```python
from build123d import *

# Parameters (mm, degrees)
SKETCH1_R           = 40
BOSS_EXTRUDE1_DEPTH = 25
SKETCH2_R           = 38
CUT_EXTRUDE1_DEPTH  = 2
SKETCH3_R           = 37
CUT_EXTRUDE2_DEPTH  = 21.5
SKETCH4_W           = 12.5
SKETCH4_H           = 11.5
CUT_EXTRUDE3_DEPTH  = 41
SKETCH5_R           = 1.05
CUT_EXTRUDE4_DEPTH  = 24
SKETCH6_W           = 4.251934594
SKETCH6_H           = 15.745280186
CUT_EXTRUDE5_DEPTH  = 1.2
SKETCH7_R           = 3.3
SKETCH7_R_2         = 1.5
BOSS_EXTRUDE2_DEPTH = 2.8
FILLET1_R           = 1
SKETCH9_R           = 4.75
SKETCH9_R_2         = 3.25
BOSS_EXTRUDE3_DEPTH = 6.4
SKETCH10_R          = 8
SKETCH10_R_2        = 3
BOSS_EXTRUDE4_DEPTH = 15.5
FILLET3_R           = 4


with BuildPart() as part:
    # Sketch1 → Boss-Extrude1 (new body)
    with BuildSketch(Plane(origin=(0, 0, 0), x_dir=(1, 0, 0), z_dir=(0, 1, 0))):
        with Locations(Location((0, 0, 0), (0, 0, 270))):  # turned: the seam where the file's is
            Circle(SKETCH1_R)
    extrude(amount=-BOSS_EXTRUDE1_DEPTH)

    # Sketch2 → Cut-Extrude1 (cut)
    with BuildSketch(Plane(origin=(0, 0, 0), x_dir=(1, 0, 0), z_dir=(0, 1, 0))):
        with Locations(Location((0, 0, 0), (0, 0, 270))):  # turned: the seam where the file's is
            Circle(SKETCH2_R)
    extrude(amount=-CUT_EXTRUDE1_DEPTH, mode=Mode.SUBTRACT)

    # Sketch3 → Cut-Extrude2 (cut)
    with BuildSketch(Plane.XZ.offset(25)):
        with Locations(Location((0, 0, 0), (0, 0, 270))):  # turned: the seam where the file's is
            Circle(SKETCH3_R)
    extrude(amount=-CUT_EXTRUDE2_DEPTH, mode=Mode.SUBTRACT)

    # Sketch4 → Cut-Extrude3 (cut, through all)
    with BuildSketch(Plane(origin=(0, 0, 0), x_dir=(0, 0, -1), z_dir=(1, 0, 0))):
        with Locations((0, -13.95)):
            Rectangle(SKETCH4_W, SKETCH4_H)
    extrude(amount=-CUT_EXTRUDE3_DEPTH, mode=Mode.SUBTRACT)

    # Sketch5 → Cut-Extrude4 (cut, through all)
    with BuildSketch(Plane(origin=(0, -2, 0), x_dir=(1, 0, 0), z_dir=(0, 1, 0))):
        with Locations(Location((-15.203530433, 3.732709011, 0), (0, 0, 270))):  # turned: the seam where the file's is
            Circle(SKETCH5_R)
        with Locations(Location((-15.203530433, 1.192709011, 0), (0, 0, 270))):  # turned: the seam where the file's is
            Circle(SKETCH5_R)
        with Locations(Location((-15.203530433, -1.347290989, 0), (0, 0, 270))):  # turned: the seam where the file's is
            Circle(SKETCH5_R)
        with Locations(Location((-15.203530433, -3.887290989, 0), (0, 0, 270))):  # turned: the seam where the file's is
            Circle(SKETCH5_R)
    extrude(amount=-CUT_EXTRUDE4_DEPTH, mode=Mode.SUBTRACT)

    # Sketch6 → Cut-Extrude5 (cut)
    with BuildSketch(Plane.XZ.offset(3.5)):
        with Locations((-15.203530433, 0.077290989)):
            Rectangle(SKETCH6_W, SKETCH6_H)
    extrude(amount=-CUT_EXTRUDE5_DEPTH, mode=Mode.SUBTRACT)

    # Sketch7 → Boss-Extrude2 (add)
    with BuildSketch(Plane.XZ.offset(3.5)):
        with Locations(Location((-22.143981065, 6.938197018, 0), (0, 0, 90))):  # turned: the seam where the file's is
            Circle(SKETCH7_R)
        with Locations(Location((-22.143981065, 6.938197018, 0), (0, 0, 270))):  # turned: the seam where the file's is
            Circle(SKETCH7_R_2, mode=Mode.SUBTRACT)
        with Locations(Location((-22.41620863, -6.284446249, 0), (0, 0, 90))):  # turned: the seam where the file's is
            Circle(SKETCH7_R)
        with Locations(Location((-22.41620863, -6.284446249, 0), (0, 0, 270))):  # turned: the seam where the file's is
            Circle(SKETCH7_R_2, mode=Mode.SUBTRACT)
    extrude(amount=BOSS_EXTRUDE2_DEPTH)

    # Fillet1
    fillet1_edges = [part.edges().sort_by_distance(p)[0] for p in [
        (-22.143981065, -3.5, 3.638197018),
    ]]
    fillet(fillet1_edges, radius=FILLET1_R)

    # Sketch9 → Boss-Extrude3 (add)
    with BuildSketch(Plane.XZ.offset(3.5)):
        with Locations(Location((0, 25, 0), (0, 0, 90))):  # turned: the seam where the file's is
            Circle(SKETCH9_R)
        with Locations(Location((0, 25, 0), (0, 0, 270))):  # turned: the seam where the file's is
            Circle(SKETCH9_R_2, mode=Mode.SUBTRACT)
        with Locations(Location((0, -25, 0), (0, 0, 90))):  # turned: the seam where the file's is
            Circle(SKETCH9_R)
        with Locations(Location((0, -25, 0), (0, 0, 90))):  # turned: the seam where the file's is
            Circle(SKETCH9_R_2, mode=Mode.SUBTRACT)
    extrude(amount=BOSS_EXTRUDE3_DEPTH)

    # Sketch10 → Boss-Extrude4 (add)
    with BuildSketch(Plane.XZ.offset(3.5)):
        with Locations(Location((0, 0, 0), (0, 0, 90))):  # turned: the seam where the file's is
            Circle(SKETCH10_R)
        with Locations(Location((0, 0, 0), (0, 0, 90))):  # turned: the seam where the file's is
            Circle(SKETCH10_R_2, mode=Mode.SUBTRACT)
    extrude(amount=BOSS_EXTRUDE4_DEPTH)

    # Fillet3
    fillet3_edges = [part.edges().sort_by_distance(p)[0] for p in [
        (0, -3.5, -8),
    ]]
    fillet(fillet3_edges, radius=FILLET3_R)


solid = part.part
```
CAD build for the part. Positions are in the model's coordinates, mm. A direction names the side the tool comes from. Coordinates: 2 decimals unless noted, no trailing zeros. Order: outer loops, then holes, each group sorted by start corner. A loop starts at its lowest first (then second) coordinate and runs counter-clockwise, first axis right, second up. Notation, with made-up numbers: M -7.5,1 L -2.5,1 A17 ccw -2.5,8 Z; hole C -35.75,48.25 d7. An arc over 180 degrees is marked long. Write each question's results on one line, items separated by ' | '. Start each with the question number.
Q1. Cut at B-B (z = 25). List the corners of the cut face in (x, y).
Q2. Cut at A-A (y = -13.75). List the corners of the cut face in (x, z), then the cut area to 3 significant figures.
Q3. Cut at D-D (x = -31). List the corners of the cut face in (y, z).
Q4. Cut at C-C (y = -23.25). List the corners of the cut face in (x, z).
Q5. Which spindle directions (+Z, -Z, +X, -X, +Y, -Y) get a long thin tool onto all of the face, cutting with end or side? Do faces 1 (the flat face through (-38, -14, 6.25)), 2 (the cylindrical face through (-25.416, -5.387, 6.509)), 3 (the cylindrical face through (-15.16, -2.15, 0.3)). Say none if no direction does.
Q6. Drill centre lines: probe 1 along X at (y, z) = (-6.5, 25); probe 2 along X at (y, z) = (-11.75, -1.5); probe 3 along X at (y, z) = (-16, 2). Where is each one in solid material? Low to high. Write a range as from..to.
Q7. Flat gauge pins, fed straight in: P1, Ø4, axis at y = -11, z = 9, coming from the -X side; P2, Ø3.5, axis at x = -22.42, z = -6.28, coming from the +Y side; P3, Ø2, axis at x = -6.5, y = -15, coming from the -Z side. Where does each tip first touch, or does it go through?
Q8. Pull direction Z, two halves, no side cores. Call faces 4 (the cylindrical face through (-24.647, -4.88, -8.717)), 5 (the cylindrical face through (-39.05, -12.32, -8.67)), 6 (the flat face through (-35.4, -25, 11.7)): +Z half, -Z half, draft (parallel to the pull), parting line (faces both ways), or undercut.
Found:
1) outline: M -31.22,-25 L -27.28,-25 L -27.28,-3.5 L -4.75,-3.5 L -4.75,-9.9 L -3.25,-9.9 L -3.25,-3.5 L 3.25,-3.5 L 3.25,-9.9 L 4.75,-9.9 L 4.75,-3.5 L 27.28,-3.5 L 27.28,-25 L 31.22,-25 L 31.22,0 L 28.62,0 L 28.62,-2 L -28.62,-2 L -28.62,0 L -31.22,0 Z
2) outline: M -39.51,-6.25 A40 ccw long -39.51,6.25 L -36.47,6.25 A37 cw long -36.47,-6.25 Z; C 0,0 d16; hole C 0,0 d6 | area: 861 mm²
3) outline: M -25,-25.28 L 0,-25.28 L 0,-21.98 L -2,-21.98 L -2,21.98 L 0,21.98 L 0,25.28 L -25,25.28 L -25,20.2 L -3.5,20.2 L -3.5,-20.2 L -25,-20.2 Z
4) outline: C 0,0 d80; hole C 0,0 d74
5) face 1: -X | face 2: -Y | face 3: +Y, -Y
6) probe 1: -31.22..-27.28, -4.75..-3.25, 3.25..4.75, 27.28..31.22 | probe 2: -7.86..-2.6, 2.6..7.86, 36.97..39.97 | probe 3: -7.75..-2.24, 2.24..7.75, 36.95..39.95
7) P1: x = -39.38 | P2: y = -2 | P3: z = -39.62
8) face 4: undercut | face 5: parting line | face 6: draft
